```python
from build123d import *

# Parameters (mm, degrees)
EXTRUDE_1_DEPTH     = 6
SKETCH_2_W          = 19
SKETCH_2_H          = 28
CUT_EXTRUDE_1_DEPTH = 6
FILLET_2_R          = 2
FILLET_3_R          = 2
SKETCH_3_R          = 1.5
CUT_EXTRUDE_2_DEPTH = 6
FILLET_4_R          = 3
FILLET_5_R          = 0.5
SKETCH_4_R          = 1.5
CUT_EXTRUDE_3_DEPTH = 14
FILLET_6_R          = 2


with BuildPart() as part:
    # 草图1 → 凸台-拉伸1 (new body)
    with BuildSketch(Plane.XY):
        with BuildLine():
            Line((12.5, 3), (24, 3))
            Line((24, 3), (24, 0))
            Line((24, 0), (-24, 0))
            Line((-24, 0), (-24, 3))
            Line((-24, 3), (-12.5, 3))
            Line((-12.5, 3), (-12.5, 44))
            ThreePointArc((-12.5, 44), (-10.458250332, 50.846531969), (-5, 55.456439237))
            Line((-5, 55.456439237), (-5, 64))
            Line((-5, 64), (-2.5, 64))
            Line((-2.5, 64), (-2.5, 53.16515139))
            ThreePointArc((-2.5, 53.16515139), (0, 34.5), (2.5, 53.16515139))
            Line((2.5, 53.16515139), (2.5, 64))
            Line((2.5, 64), (5, 64))
            Line((5, 64), (5, 55.456439237))
            ThreePointArc((5, 55.456439237), (10.458250332, 50.846531969), (12.5, 44))
            Line((12.5, 44), (12.5, 3))
        make_face()
    extrude(amount=EXTRUDE_1_DEPTH)

    # 草图2 → 切除-拉伸1 (cut)
    with BuildSketch(Plane.XY.offset(6)):
        with Locations((0, 17)):
            Rectangle(SKETCH_2_W, SKETCH_2_H)
    extrude(amount=-CUT_EXTRUDE_1_DEPTH, mode=Mode.SUBTRACT)

    # 圆角2
    fillet_2_edges = [part.edges().sort_by_distance(p)[0] for p in [
        (-9.5, 3, 3),
        (-9.5, 31, 3),
        (9.5, 31, 3),
        (9.5, 3, 3),
    ]]
    fillet(fillet_2_edges, radius=FILLET_2_R)

    # 圆角3
    fillet_3_edges = [part.edges().sort_by_distance(p)[0] for p in [
        (12.5, 3, 3),
        (-12.5, 3, 3),
    ]]
    fillet(fillet_3_edges, radius=FILLET_3_R)

    # 草图3 → 切除-拉伸2 (cut)
    with BuildSketch(Plane.XZ):
        with Locations(Location((-19, 3, 0), (0, 0, 270))):
            Circle(SKETCH_3_R)
        with Locations(Location((19, 3, 0), (0, 0, 270))):
            Circle(SKETCH_3_R)
    extrude(amount=-CUT_EXTRUDE_2_DEPTH, mode=Mode.SUBTRACT)

    # 圆角4
    fillet_4_edges = [part.edges().sort_by_distance(p)[0] for p in [
        (5, 55.456439237, 3),
        (-5, 55.456439237, 3),
    ]]
    fillet(fillet_4_edges, radius=FILLET_4_R)

    # 圆角5
    fillet_5_edges = [part.edges().sort_by_distance(p)[0] for p in [
        (5, 64, 3),
        (24, 3, 3),
        (24, 0, 3),
        (-24, 0, 3),
        (-24, 3, 3),
        (-5, 64, 3),
    ]]
    fillet(fillet_5_edges, radius=FILLET_5_R)

    # 草图4 → 切除-拉伸3 (cut)
    with BuildSketch(Plane.ZY.offset(5)):
        with Locations((3, 60)):
            Circle(SKETCH_4_R)
    extrude(amount=-CUT_EXTRUDE_3_DEPTH, mode=Mode.SUBTRACT)

    # 圆角6
    fillet_6_edges = [part.edges().sort_by_distance(p)[0] for p in [
        (2.5, 53.16515139, 3),
        (-2.5, 53.16515139, 3),
    ]]
    fillet(fillet_6_edges, radius=FILLET_6_R)


solid = part.part
```
CAD build for the part. Positions are in the model's coordinates, mm. A direction names the side the tool comes from. Give positions to 0.01 mm unless a question says otherwise; leave off trailing zeros. Write each loop counter-clockwise with the first axis right and the second up, starting at its lowest first coordinate (ties: lowest second). Pieces come first, ordered by that corner, then holes. Notation, with made-up numbers: M 38,53.25 L 62,53.25 A19 cw 62,85.25 Z; hole C 25.5,0.25 d10. An arc over 180 degrees is marked long. Return JSON: item names as keys, results as strings. Group by question number.
(1) Drill centre lines: L1, parallel to X at y = 20.5, z = 5.35; L2, parallel to Y at x = -4.5, z = 3; L3, parallel to Y at x = -3.7, z = 3. Where is each one in solid material? Low to high. Write a range as [from, to].
(2) Band-saw the part on A-A (x = 0). Give the cut face in (y, z).
(3) Band-saw the part on D-D (y = 60). Give the cut face in (x, z), and give its area (3 significant figures).
(4) Mould opens along Y. For faces 6 (the face through (2.823, 53.493, 3.042)), 7 (the face through (-12.5, 24, 3)), 8 (the face through (-4, 64, 3)) say: pulls with the +Y half, pulls with the -Y half, needs draft (parallel to the pull), parting line crosses it, or undercut.
(5) Band-saw the part on C-C (z = 3). State how many separate pieces and enclosed holes the cut face has, and give its area (3 significant figures).
(6) Flat gauge pins, fed straight in: pin 1 Ø1.8 at (y, z) = (15, 3) entering from +X; pin 2 Ø1.8 at (x, z) = (-18.5, 3.5) entering from +Y; pin 3 Ø3.5 at (y, z) = (60, 3) entering from +X; pin 4 Ø17 at (x, y) = (0, 44) entering from -Z. Where does each tip first touch, or does it go through?
(7) Band-saw the part on B-B (y = 19). Give the cut face in (x, z), and give its area (3 significant figures).
(8) 3-axis set-ups, long thin cutter, end or side, ignore diameter. For faces 1 (the face through (2.5, 58, 3)), 2 (the face through (5, 62, 3)), 3 (the face through (-2.84, 53.47, 3.04)), 4 (the face through (-20.1, 3, 1.6)), 5 (the face through (0, 32, 0)): which of +Z, -Z, +X, -X, +Y, -Y reach the whole face in a straight line?
Entries:
{
 "1": {"L1": "x = [-12.5, -9.5], [9.5, 12.5]", "L2": "y = [0, 3], [31, 35.63], [52.37, 58.5], [61.5, 64]", "L3": "y = [0, 3], [31, 35.25], [52.75, 58.5], [61.5, 64]"},
 "2": {"outline": "M 0,0 L 3,0 L 3,6 L 0,6 Z; M 31,0 L 34.5,0 L 34.5,6 L 31,6 Z"},
 "3": {"outline": "M -5,0 L -2.5,0 L -2.5,1.5 L -5,1.5 Z; M -5,4.5 L -2.5,4.5 L -2.5,6 L -5,6 Z; M 2.5,0 L 5,0 L 5,1.5 L 2.5,1.5 Z; M 2.5,4.5 L 5,4.5 L 5,6 L 2.5,6 Z", "area": "15.0 mm^2"},
 "4": {"face 6": "undercut", "face 7": "needs draft", "face 8": "pulls with the +Y half"},
 "5": {"separate pieces": "5", "enclosed holes": "1", "area": "596 mm^2"},
 "6": {"pin 1": "stops at x = 12.5", "pin 2": "stops at y = 3", "pin 3": "stops at x = 5", "pin 4": "passes through"},
 "7": {"outline": "M -12.5,0 L -9.5,0 L -9.5,6 L -12.5,6 Z; M 9.5,0 L 12.5,0 L 12.5,6 L 9.5,6 Z", "area": "36.0 mm^2"},
 "8": {"face 1": "+Z, -Z, +Y", "face 2": "+Z, -Z, +X, +Y", "face 3": "+Z, -Z", "face 4": "+Z, -Z, -X, +Y", "face 5": "-Z, +X, -X, +Y, -Y"}
}
